Job drawing, mm, ordinate dimensions from the low corner. One solid piece. Round coordinates to 2 decimals unless told otherwise and drop trailing zeros. Loops run counter-clockwise (first coordinate to the right, second up) from the corner with the lowest first, then second, coordinate; pieces in that order, holes last.
1) Drop a flat-ended pin along its axis: P1, Ø5.5, axis at x = 80, z = 100, coming from the +Y side. Give the stop position or say it passes through.
2) Band-saw the part on B-B, the plane z = 125.46. Write the cut outline in (x, y), then the cut area to 3 significant figures.
3) Mould opens along Z. For the marked faces 1 and 2 say: +Z half, -Z half, draft (parallel to the pull), parting line (faces both ways), or undercut.
4) Band-saw the part on C-C, the plane x = 19. Write the cut outline in (y, z), then the cut area to 3 significant figures.
5) Probe line 1 (X direction, y = 12.6, z = 80.46); line 2 (Y direction, x = 65.5, z = 16); line 3 (X direction, y = 11.25, z = 95). List the from-to ranges inside material, lowest first.
6) Band-saw the part on D-D, the plane z = 158. Write the cut outline in (x, y).
7) Band-saw the part on A-A, the plane y = 13. State how many separate pieces and enclosed holes the cut face has, then the cut area to 3 significant figures.
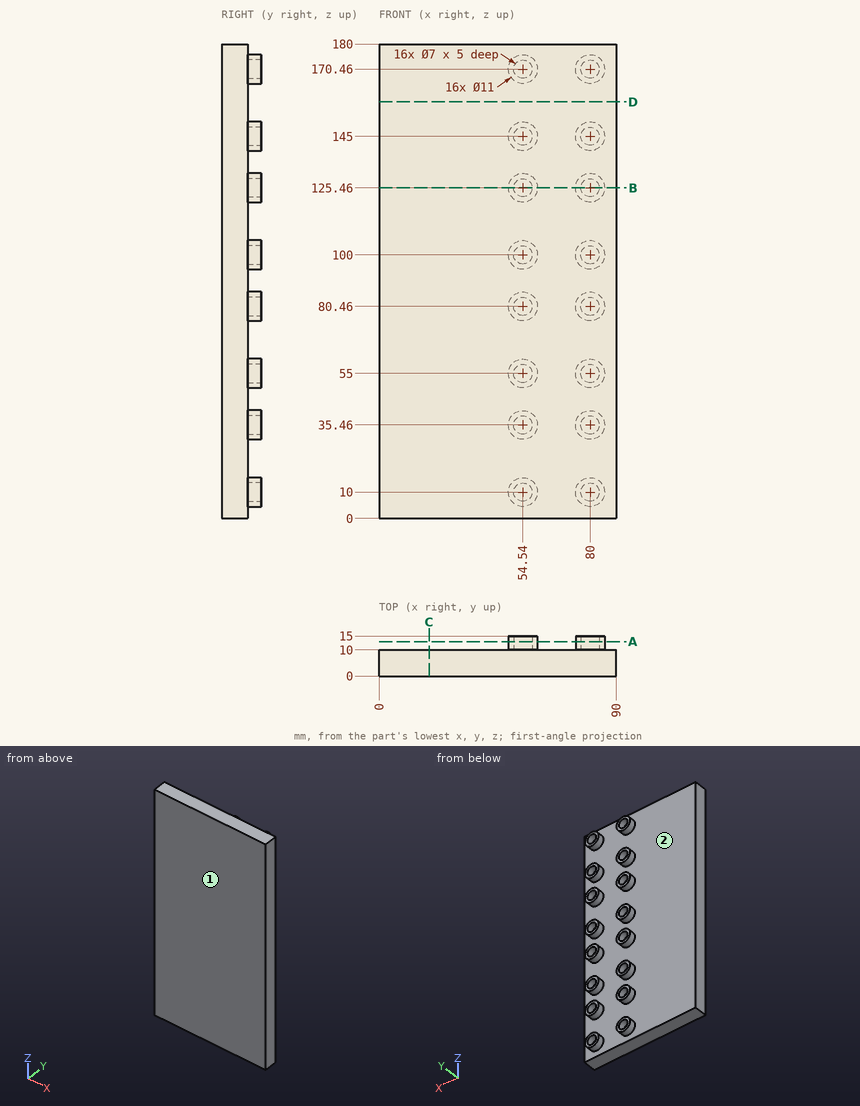
Reported:
1. P1: stops at y = 10
2. outline: (0, 0) - (90, 0) - (90, 10) - (85.5, 10) - (85.5, 15) - (83.5, 15) - (83.5, 10) - (76.5, 10) - (76.5, 15) - (74.5, 15) - (74.5, 10) - (60.04, 10) - (60.04, 15) - (58.04, 15) - (58.04, 10) - (51.04, 10) - (51.04, 15) - (49.04, 15) - (49.04, 10) - (0, 10) - close
2. area: 940 mm2
3. face 1: draft
3. face 2: undercut
4. outline: (0, 0) - (10, 0) - (10, 180) - (0, 180) - close
4. area: 1,800 mm2
5. line 1: x = 49.04 to 51.04, 58.04 to 60.04, 74.5 to 76.5, 83.5 to 85.5
5. line 2: y = 0 to 10
5. line 3: x = 52.25 to 56.83, 77.71 to 82.29
6. outline: (0, 0) - (90, 0) - (90, 10) - (0, 10) - close
7. separate pieces: 16
7. enclosed holes: 16
7. area: 905 mm2
